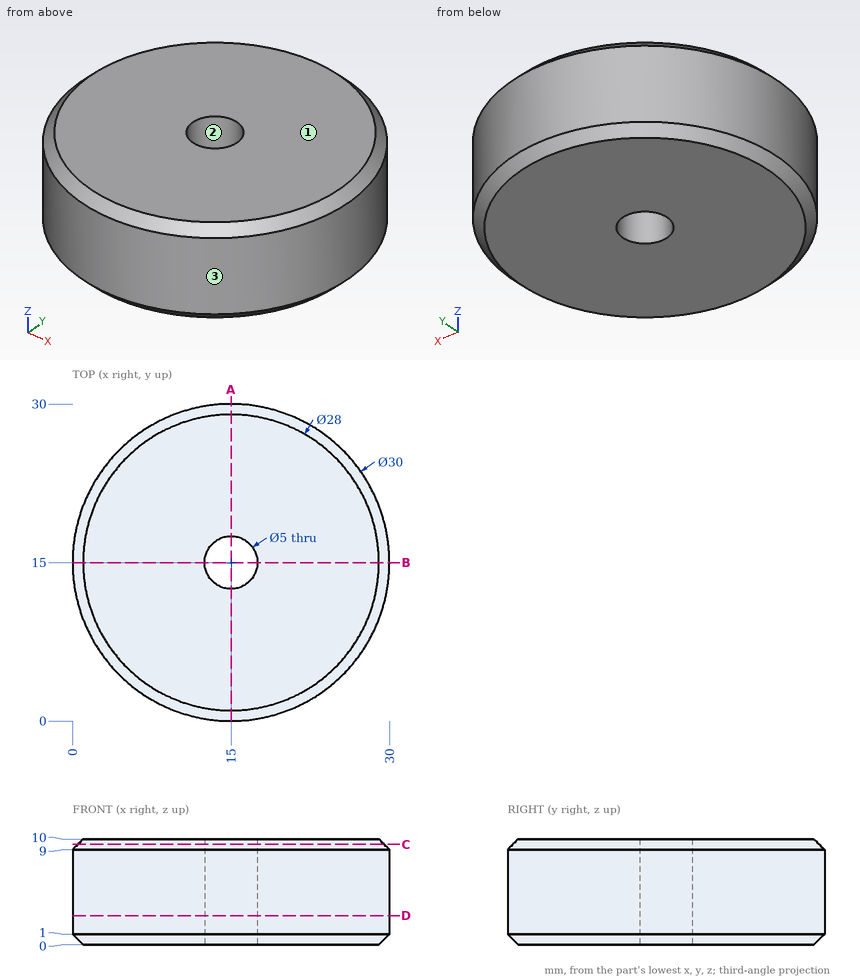
Drawing for the job (mm, zero at the part's lowest x, y, z). Give positions to 0.01 mm unless a question says otherwise; leave off trailing zeros. Write each loop counter-clockwise with the first axis right and the second up, starting at its lowest first coordinate (ties: lowest second). Pieces come first, ordered by that corner, then holes. Notation, with made-up numbers: M -21,64 L 33,64 A21 ccw 33,89 Z; hole C 74.25,-39 d2. An arc over 180 degrees is marked long. Return JSON: item names as keys, results as strings. Group by question number.
(1) Band-saw the part on C-C (z = 9.5). Give the cut face in (x, y), and give its area (3 significant figures).
(2) Flat gauge pins, fed straight in: pin 1 Ø2 at (y, z) = (3, 7) entering from +X; pin 2 Ø6 at (y, z) = (24.5, 5) entering from +X; pin 3 Ø1.5 at (x, z) = (23.5, 5) entering from +Y. Where does each tip first touch, or does it go through?
(3) Band-saw the part on D-D (z = 2.75). Give the cut face in (x, y).
(4) Mould opens along X. For the marked faces 1, 2 and 3 say: pulls with the +X half, pulls with the -X half, needs draft (parallel to the pull), parting line crosses it, or undercut.
(5) Band-saw the part on A-A (x = 15). Give the cut face in (y, z), and give its area (3 significant figures).
(6) Drill centre lines: L1, parallel to Y at x = 15, z = 3; L2, parallel to X at y = 9, z = 9.25; L3, parallel to Y at x = 15.5, z = 6.75. Where is each one in solid material? Low to high. Write a range as [from, to].
Entries:
{
 "1": {"outline": "C 15,15 d29; hole C 15,15 d5", "area": "641 mm^2"},
 "2": {"pin 1": "stops at x = 25.2", "pin 2": "stops at x = 28.52", "pin 3": "stops at y = 27.84"},
 "3": {"outline": "C 15,15 d30; hole C 15,15 d5"},
 "4": {"face 1": "needs draft", "face 2": "undercut", "face 3": "parting line crosses it"},
 "5": {"outline": "M 0,1 L 1,0 L 12.5,0 L 12.5,10 L 1,10 L 0,9 Z; M 17.5,0 L 29,0 L 30,1 L 30,9 L 29,10 L 17.5,10 Z", "area": "248 mm^2"},
 "6": {"L1": "y = [0, 12.5], [17.5, 30]", "L2": "x = [1.53, 28.47]", "L3": "y = [0.01, 12.55], [17.45, 29.99]"}
}
